Could you check a few things on this model? Use its own coordinates, in mm. Face numbers are marked on the shaded views. Coordinates: 2 decimals unless noted, no trailing zeros. Write each loop counter-clockwise with the first axis right and the second up, starting at its lowest first coordinate (ties: lowest second). Pieces come first, ordered by that corner, then holes. Notation, with made-up numbers: (13.25, 48.5) - (22.25, 48.5) arc R24 cw to (22.25, 73.5) - close; hole circle Ø11 at (-22, -5). An arc over 180 degrees is marked (long way). Answer as a JSON object with one key per item and string values. Group by question number.
1) Will these pins go through, and if not, where does the flat tip stop? pin 1 Ø3 at (x, z) = (-1.5, 9.5) entering from +Y; pin 2 Ø3 at (y, z) = (9.5, 0) entering from +X; pin 3 Ø1.4 at (x, y) = (4.6, 0) entering from +Z.
2) If we section it at C-C (x = 0.25): Write out the boundary of the cut face in (y, z).
3) We'd pull the mould along Y, two halves only. Please class the marked faces 1, 2 and 3: released by +Y, released by -Y, zero draft, split by the parting line, or undercut.
4) If we section it at A-A (y = 0): Write out the boundary of the cut face in (x, z), plus the area to 3 significant figures.
5) If we section it at D-D (y = -9.5): Write out the boundary of the cut face in (x, z), plus the area to 3 significant figures.
6) If we section it at B-B (y = 4.75): Write out the boundary of the cut face in (x, z), plus the area to 3 significant figures.
7) Please list where these lines run through material, in increasing order: line 1 along X through (y, z) = (0, 3.55); line 2 along Z through (x, y) = (1.5, 0); line 3 along Y through (x, z) = (1, -1).
```python
from build123d import *

# Parameters (mm, degrees)
F3_D            = 2.4
F3_COPIES_COUNT = 6
F6_D            = 2.4
F6_DEPTH        = 12.7
F6_START        = 0.0568201
F6_TIP          = 0.7210327428
F9_D            = 2.4
F9_DEPTH        = 5
F9_START        = 0.1212247
F9_TIP          = 0.7210327428


# Not quite as in the source:
# - a pattern or mirror of a feature is missing from the dataset's text; its kind, count and spacing are read off the source's solid


with BuildPart() as f1:
    # F0 (on Front) → F1 (revolve)
    with BuildSketch(Plane.XZ):
        Polygon((-2.5, 12.7), (-2.5, 3), (6.7, 3), (6.7, 6), (2.5, 6), (2.5, 12.7), align=None)
    revolve(axis=Axis((2.1, 0, 0), (1, 0, 0)))

    # F3 (through all)
    with Locations(Plane.YZ.offset(2.5)):
        with Locations((4.75, 8.227241336)):
            f3 = Hole(F3_D / 2)

    # F3_copies: F3 ×6 about axis
    f3_copies_axis = Axis((0, 0, 0), (1, 0, 0))
    for i in range(1, F3_COPIES_COUNT):
        add(f3.rotate(f3_copies_axis, i * 360 / F3_COPIES_COUNT), mode=Mode.SUBTRACT)

    # F6
    # its depths count from where the whole tool has entered the part; down to there all is cleared
    with Locations(Plane.XY.offset(12.7).offset(-F6_START)):
        with Locations((0, 0)):
            Hole(F6_D / 2, depth=F6_DEPTH)
            with Locations((0, 0, -(F6_DEPTH + F6_TIP / 2))):  # 118° drill point
                Cone(0, F6_D / 2, F6_TIP, mode=Mode.SUBTRACT)

    # F9
    # its depths count from where the whole tool has entered the part; down to there all is cleared
    with Locations(Plane.XY.offset(6).offset(-F9_START)):
        with Locations((4.6, 0)):
            Hole(F9_D / 2, depth=F9_DEPTH)
            with Locations((0, 0, -(F9_DEPTH + F9_TIP / 2))):  # 118° drill point
                Cone(0, F9_D / 2, F9_TIP, mode=Mode.SUBTRACT)


solid = f1.part
```
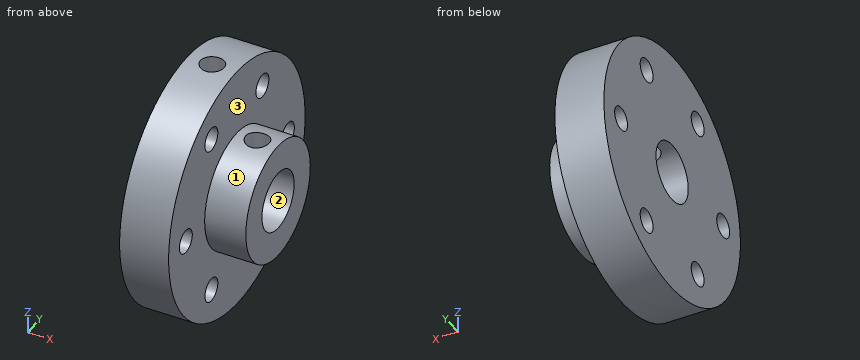
Here are the results:
{
 "1": {"pin 1": "stops at y = 9.86", "pin 2": "stops at x = 2.5", "pin 3": "stops at z = -2.92"},
 "2": {"outline": "(-1.17, 2.76) - (-1.17, 12.65) arc R12.7 ccw (long way) to (1.17, 12.65) - (1.17, 2.76) arc R3 cw (long way) to start; hole circle Ø2.4 at (-9.5, 0); hole circle Ø2.4 at (-4.75, -8.23); hole circle Ø2.4 at (-4.75, 8.23); hole circle Ø2.4 at (4.75, -8.23); hole circle Ø2.4 at (4.75, 8.23); hole circle Ø2.4 at (9.5, 0)"},
 "3": {"face 1": "split by the parting line", "face 2": "undercut", "face 3": "zero draft"},
 "4": {"outline": "(-2.5, -12.7) - (2.5, -12.7) - (2.5, -6) - (6.7, -6) - (6.7, -3) - (-2.5, -3) - close; (-2.5, 3) - (-1.2, 3) - (-1.2, 12.7) - (-2.5, 12.7) - close; (1.2, 3) - (3.4, 3) - (3.4, 6) - (2.5, 6) - (2.5, 12.7) - (1.2, 12.7) - close; (5.8, 3) - (6.7, 3) - (6.7, 6) - (5.8, 6) - close", "area": "91.7 mm²"},
 "5": {"outline": "(-2.5, -8.43) - (2.5, -8.43) - (2.5, -1.2) - (-2.5, -1.2) - close; (-2.5, 1.2) - (2.5, 1.2) - (2.5, 8.43) - (-2.5, 8.43) - close", "area": "72.3 mm²"},
 "6": {"outline": "(-2.5, -11.78) - (2.5, -11.78) - (2.5, -9.43) - (-2.5, -9.43) - close; (-2.5, -7.03) - (2.5, -7.03) - (2.5, -3.67) - (6.7, -3.67) - (6.7, 3.67) - (2.5, 3.67) - (2.5, 7.03) - (-2.5, 7.03) - close; (-2.5, 9.43) - (2.5, 9.43) - (2.5, 11.78) - (-2.5, 11.78) - close", "area": "125 mm²"},
 "7": {"line 1": "x = -2.5 to -1.2, 1.2 to 3.4, 5.8 to 6.7", "line 2": "z = -12.7 to -3, 3 to 12.7", "line 3": "y = -12.66 to -10.16, -8.84 to -2.83, 2.83 to 8.84, 10.16 to 12.66"}
}
